Geometry check sheet. Reference: the model listing, model coordinates, mm. Round coordinates to 2 decimals unless told otherwise and drop trailing zeros. Order: outer loops, then holes, each group sorted by start corner. A loop starts at its lowest first (then second) coordinate and runs counter-clockwise, first axis right, second up. Notation, with made-up numbers: (37.5, 39.5) - (65.5, 39.5) arc R21 ccw to (65.5, 64.5) - close; hole circle Ø8 at (-27.75, 19.5). An arc over 180 degrees is marked (long way). Return JSON: item names as keys, results as strings. Group by question number.
Q1. Sectioned sample at C-C, the plane z = -78. Record the cut outline in (x, y).
Q2. Sectioned sample at B-B, the plane x = 112.5. Record the cut outline in (y, z), then the cut area to 3 significant figures.
Q3. Material ranges on line 1 along Z through (x, y) = (172, 0.35); line 2 along Z through (x, y) = (86.5, 0.4); line 3 along Z through (x, y) = (69, 0.6), recorded low to high.
Q4. Sectioned sample at A-A, the plane z = -61.5. Record the cut outline in (x, y).
Q5. Sectioned sample at D-D, the plane y = 0.15. Give the number of separate pieces and of enclosed holes in the cut face, then the cut area to 3 significant figures.
```python
from build123d import *

# Parameters (mm, degrees)
SKETCH1_W           = 239.2
SKETCH1_H           = 119.2
BOSS_EXTRUDE1_DEPTH = 0.8
FILLET2_R           = 16
FILLET3_R           = 4


with BuildPart() as part:
    # Sketch1 → Boss-Extrude1 (new body)
    with BuildSketch(Plane(origin=(0, 0, 0), x_dir=(1, 0, 0), z_dir=(0, 1, 0))):
        with Locations((119.6, 59.6)):
            Rectangle(SKETCH1_W, SKETCH1_H)
        Polygon((10, 107.2), (60.440329218, 59.6), (10, 12), align=None, mode=Mode.SUBTRACT)
        Polygon((12, 109.2), (113, 109.2), (62.5, 61.54368932), align=None, mode=Mode.SUBTRACT)
        Polygon((12, 10), (113, 10), (62.5, 57.65631068), align=None, mode=Mode.SUBTRACT)
        Polygon((115, 107.2), (115, 12), (64.559670782, 59.6), align=None, mode=Mode.SUBTRACT)
        Polygon((127, 109.2), (227.2, 109.2), (177.1, 61.551076321), align=None, mode=Mode.SUBTRACT)
        Polygon((125, 107.2), (125, 12), (175.048559671, 59.6), align=None, mode=Mode.SUBTRACT)
        Polygon((127, 10), (227.2, 10), (177.1, 57.648923679), align=None, mode=Mode.SUBTRACT)
        Polygon((229.2, 107.2), (229.2, 12), (179.151440329, 59.6), align=None, mode=Mode.SUBTRACT)
    extrude(amount=BOSS_EXTRUDE1_DEPTH)

    # Fillet2
    fillet2_edges = [part.edges().sort_by_distance(p)[0] for p in [
        (62.5, 0.4, -61.54368932),
        (60.440329218, 0.4, -59.6),
        (175.048559671, 0.4, -59.6),
        (177.1, 0.4, -57.648923679),
        (177.1, 0.4, -61.551076321),
        (62.5, 0.4, -57.65631068),
        (64.559670782, 0.4, -59.6),
        (179.151440329, 0.4, -59.6),
    ]]
    fillet(fillet2_edges, radius=FILLET2_R)

    # Fillet3
    fillet3_edges = [part.edges().sort_by_distance(p)[0] for p in [
        (113, 0.4, -109.2),
        (12, 0.4, -109.2),
        (10, 0.4, -12),
        (10, 0.4, -107.2),
        (125, 0.4, -107.2),
        (125, 0.4, -12),
        (227.2, 0.4, -10),
        (127, 0.4, -10),
        (227.2, 0.4, -109.2),
        (127, 0.4, -109.2),
        (113, 0.4, -10),
        (12, 0.4, -10),
        (115, 0.4, -12),
        (115, 0.4, -107.2),
        (229.2, 0.4, -12),
        (229.2, 0.4, -107.2),
    ]]
    fillet(fillet3_edges, radius=FILLET3_R)


solid = part.part
```
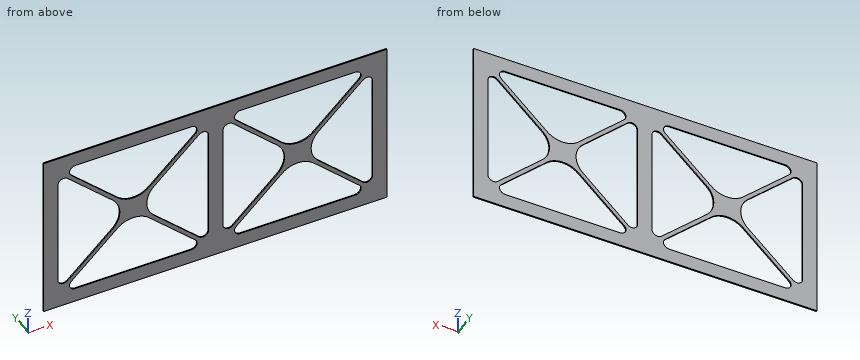
Reply:
{
 "1": {"outline": "(0, 0) - (10, 0) - (10, 0.8) - (0, 0.8) - close; (40.94, 0) - (45.06, 0) - (45.06, 0.8) - (40.94, 0.8) - close; (79.94, 0) - (84.06, 0) - (84.06, 0.8) - (79.94, 0.8) - close; (115, 0) - (125, 0) - (125, 0.8) - (115, 0.8) - close; (155.7, 0) - (159.8, 0) - (159.8, 0.8) - (155.7, 0.8) - close; (194.4, 0) - (198.5, 0) - (198.5, 0.8) - (194.4, 0.8) - close; (229.2, 0) - (239.2, 0) - (239.2, 0.8) - (229.2, 0.8) - close"},
 "2": {"outline": "(0, -119.2) - (0.8, -119.2) - (0.8, -101.63) - (0, -101.63) - close; (0, -17.57) - (0.8, -17.57) - (0.8, 0) - (0, 0) - close", "area": "28.1 mm^2"},
 "3": {"line 1": "-119.2 to -109.2, -68.47 to -50.73, -10 to 0", "line 2": "-119.2 to -109.2, -84.19 to -80.3, -38.9 to -35.01, -10 to 0", "line 3": "-119.2 to -109.2, -68.92 to -50.28, -10 to 0"},
 "4": {"outline": "(0, 0) - (10, 0) - (10, 0.8) - (0, 0.8) - close; (53.01, 0) - (71.99, 0) - (71.99, 0.8) - (53.01, 0.8) - close; (115, 0) - (125, 0) - (125, 0.8) - (115, 0.8) - close; (167.72, 0) - (186.48, 0) - (186.48, 0.8) - (167.72, 0.8) - close; (229.2, 0) - (239.2, 0) - (239.2, 0.8) - (229.2, 0.8) - close"},
 "5": {"separate pieces": "1", "enclosed holes": "8", "area": "10,100 mm^2"}
}
